Could you check a few things on this model? Use its own coordinates, in mm. A direction names the side the tool comes from. Give positions to 0.01 mm unless a question says otherwise; leave off trailing zeros. Loops run counter-clockwise (first coordinate to the right, second up) from the corner with the lowest first, then second, coordinate; pieces in that order, holes last. Notation, with made-up numbers: (71.5, 24) - (120.5, 24) arc R30 ccw to (120.5, 60) - close; hole circle Ø4 at (-6.75, 73). An arc over 180 degrees is marked (long way). Answer in a Markdown table with one row per item. Add a question column.
Autodesk Inventor part; units mm, degrees
ref_plane "YZ Plane" through (0, 0, 0) normal (1, 0, 0) x (0, 1, 0)
ref_plane "XZ Plane" through (0, 0, 0) normal (0, 1, 0) x (-1, 0, 0)
ref_plane "XY Plane" through (0, 0, 0) normal (0, 0, 1) x (1, 0, 0)
sketch "Sketch1" plane through (0, 0, 0) normal (0, 1, 0) x (-1, 0, 0)
  circle A0 centre (-8.0963, -24.7317) radius 1.5
  circle A1 centre (7.9037, -24.7317) radius 1.5
  line L0 (-11.8963, -27.0317) -> (11.2037, -27.0317)
  line L1 (11.2037, 21.8683) -> (-11.8963, 21.8683)
  line L2 (-0.3463, 7.8683) -> (-0.3463, 9.8683)
  line L3 (-2.3463, 9.8683) -> (-11.8963, 9.8683)
  line L4 (-13.8963, -29.0317) -> (13.2037, -29.0317)
  line L5 (13.2037, -29.0317) -> (13.2037, 23.8683)
  line L6 (13.2037, 23.8683) -> (-13.8963, 23.8683)
  line L7 (-13.8963, 23.8683) -> (-13.8963, -29.0317)
  line L8 (-0.3463, 7.8683) -> (-11.8963, 7.8683)
  line L9 (-11.8963, 21.8683) -> (-11.8963, 7.8683)
  line L10 (11.2037, 12.8683) -> (-0.3463, 12.8683)
  line L11 (-0.3463, 9.8683) -> (-0.3463, 12.8683)
  line L12 (-2.3463, 14.8683) -> (-2.3463, 9.8683)
  line L13 (-2.3463, 14.8683) -> (11.2037, 14.8683)
  line L14 (11.2037, -16.9317) -> (-11.8963, -16.9317)
  line L15 (-11.8963, -20.9317) -> (11.2037, -20.9317)
  line L16 (-11.8963, 7.8683) -> (-11.8963, -20.9317)
  line L17 (-11.8963, -20.9317) -> (-11.8963, -27.0317)
  line L18 (11.2037, -27.0317) -> (11.2037, 21.8683)
  point P0 (0, 0)
  point P1 (-15.2463, -4.6317)
  dimension "d0" = 2
  dimension "d12" = 6.1
extrude "Extrusion1" add sketch "Sketch1" against normal blind 2 contours A0 | A1 | L17 L15 L18 L0 | L16 L14 L18 L15 | L16 L8 L2 L11 L10 L18 L14 | L9 L3 L12 L13 L18 L10 L11 L2 L8 | L9 L1 L18 L13 L12 L3 | L7 L6 L5 L4
extrude "Extrusion2" add sketch "Sketch1" along normal blind 6
extrude "Extrusion3" add sketch "Sketch1" along normal blind 2 contours L9 L3 L12 L13 L18 L10 L11 L2 L8
extrude "Extrusion4" add sketch "Sketch1" along normal blind 3.5 contours L16 L14 L18 L15
sketch "Sketch3" plane through (13.8963, -2, 23.8683) normal (1, 0, 0) x (0, 0, -1)
  arc A0 (30.6, 9.1) -> (28.5, 11.2) centre (28.5, 9.1) ccw
  arc A1 (21.8, 11.2) -> (19.7, 9.1) centre (21.8, 9.1) ccw
  line L0 (20.7, 8.1) -> (20.7, 9.1)
  line L1 (20.7, 8.1) -> (20.7, 9.1)
  line L2 (20.7, 9.1) -> (20.7, 8.1)
  arc A2 (21.8, 10.2) -> (20.7, 9.1) centre (21.8, 9.1) ccw
  line L3 (0, 0) -> (0, 8)
  line L4 (29.6, 9.1) -> (29.6, 8.1)
  line L5 (29.6, 8.1) -> (29.6, 9.1)
  line L6 (28.5, 10.2) -> (21.8, 10.2)
  arc A3 (29.6, 9.1) -> (28.5, 10.2) centre (28.5, 9.1) ccw
  line L7 (30.6, 8.1) -> (30.6, 9.1)
  line L8 (29.6, 8.1) -> (29.6, 9.1)
  arc A4 (28.5, 6) -> (30.6, 8.1) centre (28.5, 8.1) ccw
  line L9 (28.5, 11.2) -> (21.8, 11.2)
  line L10 (21.8, 10.2) -> (28.5, 10.2)
  line L11 (28.5, 10.2) -> (21.8, 10.2)
  line L12 (21.8, 7) -> (28.5, 7)
  line L13 (28.5, 7) -> (21.8, 7)
  line L14 (21.8, 6) -> (28.5, 6)
  line L15 (19.7, 9.1) -> (19.7, 8.1)
  arc A5 (20.7, 8.1) -> (21.8, 7) centre (21.8, 8.1) ccw
  arc A6 (19.7, 8.1) -> (21.8, 6) centre (21.8, 8.1) ccw
  line L16 (52.9, 8) -> (52.9, 0)
  line L17 (0, 8) -> (52.9, 8)
  line L18 (52.9, 0) -> (0, 0)
  arc A7 (28.5, 7) -> (29.6, 8.1) centre (28.5, 8.1) ccw
  point P0 (23.8683, 2)
  point P1 (29.0317, 2)
  point P2 (20.7, 10.2)
  point P3 (29.6, 7)
  point P4 (30.5976, 8)
  point P5 (19.7024, 8)
  dimension "d21" = 1.1
  dimension "d22" = 1
extrude "Extrusion6" cut sketch "Sketch3" against normal blind 6 contours A4 L14 A6 L17 A5 L12 A7 | A7 L12 A5 L17
properties part number "base"
(1) I want a section at A-A on z = -14. Please give me the cut outline in (x, y), then the cut area to 3 significant figures.
(2) I want a section at C-C on x = 4.25. Please give me the cut outline in (y, z).
(3) On a 3-axis mill with a long thin cutter (end or side, diameter ignored), from which of +Z, -Z, +X, -X, +Y, -Y can I reach the whole of each face in a straight line? I mean faces 4 (the flat face through (13, 4, -1)), 5 (the flat face through (-4, 1, 14.868)), 6 (the flat face through (1, -2, -2)). Say none if no direction works.
(4) Please list where these lines run through material, in increasing order: line 1 (Z direction, x = -10.25, y = 1.75); line 2 (Z direction, x = 3.25, y = 2.25); line 3 (X direction, y = 1.25, z = 18).
(5) For pin 1 Ø3 at (x, z) = (-1, 1.5) entering from +Y; pin 2 Ø1.2 at (x, z) = (4.5, -18) entering from +Y; pin 3 Ø1 at (x, z) = (12.5, -1) entering from +Y; pin 4 Ø13 at (x, z) = (-1, 16) entering from +Y, each with a flat end and sliding along its axis, tell me the tip position at first contact or that it passes through.
(6) We'd pull the mould along X, two halves only. Please class faces 1 (the flat face through (0, 2, 23.868)), 2 (the flat face through (1, 2, -20.932)), 3 (the flat face through (13.896, 2, -2)): pulls with the +X half, pulls with the -X half, needs draft (parallel to the pull), parting line crosses it, or undercut.
(7) I want a section at B-B on y = 5. Please give me the cut outline in (x, z).
(8) I want a section at D-D on z = 8.5. Please give me the cut outline in (x, y), then the cut area to 3 significant figures.
Reported:
| question | item | result |
|---|---|---|
| 1 | outline | (-13.2, -2) - (13.9, -2) - (13.9, 6) - (11.9, 6) - (11.9, 0) - (-11.2, 0) - (-11.2, 6) - (-13.2, 6) - close |
| 1 | area | 78.2 mm² |
| 2 | outline | (-2, -29.03) - (6, -29.03) - (6, -27.03) - (0, -27.03) - (0, -20.93) - (3.5, -20.93) - (3.5, -16.93) - (0, -16.93) - (0, 7.87) - (2, 7.87) - (2, 9.87) - (0, 9.87) - (0, 21.87) - (6, 21.87) - (6, 23.87) - (-2, 23.87) - close |
| 3 | face 4 | +X, +Y |
| 3 | face 5 | +Y |
| 3 | face 6 | +Z, -Z, +X, -X, -Y |
| 4 | line 1 | -29.03 to -27.03, -20.93 to -16.93, 12.87 to 14.87, 21.87 to 23.87 |
| 4 | line 2 | -29.03 to -27.03, -20.93 to -16.93, 21.87 to 23.87 |
| 4 | line 3 | -13.2 to -11.2, 11.9 to 13.9 |
| 5 | pin 1 | y = 0 |
| 5 | pin 2 | y = 3.5 |
| 5 | pin 3 | y = 4 |
| 5 | pin 4 | y = 6 |
| 6 | face 1 | needs draft |
| 6 | face 2 | undercut |
| 6 | face 3 | pulls with the +X half |
| 7 | outline | (-13.2, -29.03) - (13.9, -29.03) - (13.9, -6.42) - (11.9, -6.42) - (11.9, -27.03) - (-11.2, -27.03) - (-11.2, 21.87) - (11.9, 21.87) - (11.9, 3.86) - (13.9, 3.86) - (13.9, 23.87) - (-13.2, 23.87) - close; circle Ø3 at (-7.9, -24.73); circle Ø3 at (8.1, -24.73) |
| 8 | outline | (-13.2, -2) - (13.9, -2) - (13.9, 6) - (11.9, 6) - (11.9, 2) - (0.35, 2) - (0.35, 0) - (-11.2, 0) - (-11.2, 6) - (-13.2, 6) - close |
| 8 | area | 101 mm² |
